from build123d import *

# Parameters (mm, degrees)
SKETCH_1_W          = 45
SKETCH_1_H          = 45
EXTRUDE_1_DEPTH     = 5
SKETCH_2_R          = 1
CUT_EXTRUDE_2_DEPTH = 5
SKETCH_3_W          = 35
SKETCH_3_H          = 5
CUT_EXTRUDE_3_DEPTH = 33.210246817
SKETCH_4_W          = 5
SKETCH_4_H          = 40
EXTRUDE_2_DEPTH     = 20


with BuildPart() as part:
    # 草圖1 → 填料-伸長1 (new body)
    with BuildSketch(Plane.XY):
        Rectangle(SKETCH_1_W, SKETCH_1_H)
    extrude(amount=EXTRUDE_1_DEPTH)

    # 草圖2 → 除料-伸長2 (cut)
    with BuildSketch(Plane(origin=(22.5, 0, 0), x_dir=(0, 0, -1), z_dir=(1, 0, 0))):
        with Locations(Location((-2.5, 20, 0), (0, 0, 90))):
            Circle(SKETCH_2_R)
    cut_extrude_2 = extrude(amount=-CUT_EXTRUDE_2_DEPTH, mode=Mode.SUBTRACT)

    # 草圖3 → 除料-伸長3 (cut, through all)
    with BuildSketch(Plane(origin=(0, 0, 0), x_dir=(-1, 0, 0), z_dir=(0, 0, -1))):
        with Locations((0, 20)):
            Rectangle(SKETCH_3_W, SKETCH_3_H)
    extrude(amount=-CUT_EXTRUDE_3_DEPTH, mode=Mode.SUBTRACT)

    # 鏡射1: 除料-伸長2 across plane
    add(cut_extrude_2.mirror(Plane(origin=(0, 0, 0), x_dir=(0, 0, 1), z_dir=(1, 0, 0))), mode=Mode.SUBTRACT)

    # 草圖4 → 填料-伸長2 (add)
    with BuildSketch(Plane(origin=(0, 0, 0), x_dir=(-1, 0, 0), z_dir=(0, 0, -1))):
        with Locations((-20, -2.5)):
            Rectangle(SKETCH_4_W, SKETCH_4_H)
    extrude_2 = extrude(amount=EXTRUDE_2_DEPTH)

    # 鏡射2: 填料-伸長2 across plane
    add(extrude_2.mirror(Plane(origin=(0, 0, 0), x_dir=(0, 0, 1), z_dir=(1, 0, 0))))


solid = part.part
Can you work these out from the model? Positions are in its coordinate system, mm. A direction names the side the tool comes from. Give positions to 0.01 mm unless a question says otherwise; leave off trailing zeros. Loops run counter-clockwise (first coordinate to the right, second up) from the corner with the lowest first, then second, coordinate; pieces in that order, holes last. Notation, with made-up numbers: (-28.5, -14) - (-16.5, -14) arc R37 cw to (-16.5, 25) - close; hole circle Ø1 at (38.5, -33.75). An arc over 180 degrees is marked (long way). Answer as a JSON object with one key per item and string values.
Q1. If I drill on L1, parallel to Z at x = -21, y = 20; L2, parallel to X at y = -18, z = -1.25; L3, parallel to Z at x = -12, y = -8.5, over which ranges is the centre line in solid material (lowest first)?
Geometry says:
{"L1": "0 to 1.5, 3.5 to 5", "L2": "-22.5 to -17.5, 17.5 to 22.5", "L3": "0 to 5"}
Q2. Imagine slicing it at D-D on y = -4. Write out the boundary of the cut face in (x, z).
Geometry says:
{"outline": "(-22.5, -20) - (-17.5, -20) - (-17.5, 0) - (17.5, 0) - (17.5, -20) - (22.5, -20) - (22.5, 5) - (-22.5, 5) - close"}
Q3. Will these pins go through, and if not, where does the flat tip stop? P1, Ø1.5, axis at x = -20, y = 20, coming from the -Z side; P2, Ø3, axis at y = 20, z = 2.5, coming from the +X side; P3, Ø5.5, axis at x = -3, z = 2, coming from the +Y side.
Geometry says:
{"P1": "z = 0", "P2": "x = 22.5", "P3": "y = 17.5"}
Q4. Imagine slicing it at B-B on y = 20. Write out the boundary of the cut face in (x, z).
Geometry says:
{"outline": "(-22.5, 0) - (-17.5, 0) - (-17.5, 1.5) - (-22.5, 1.5) - close; (-22.5, 3.5) - (-17.5, 3.5) - (-17.5, 5) - (-22.5, 5) - close; (17.5, 0) - (22.5, 0) - (22.5, 1.5) - (17.5, 1.5) - close; (17.5, 3.5) - (22.5, 3.5) - (22.5, 5) - (17.5, 5) - close"}
Q5. Imagine slicing it at C-C on z = -7.75. Write out the boundary of the cut face in (x, y), plus the area to 3 significant figures.
Geometry says:
{"outline": "(-22.5, -22.5) - (-17.5, -22.5) - (-17.5, 17.5) - (-22.5, 17.5) - close; (17.5, -22.5) - (22.5, -22.5) - (22.5, 17.5) - (17.5, 17.5) - close", "area": "400 mm²"}
Q6. Which directions (+Z, -Z, +X, -X, +Y, -Y) give clear straight access to the entire face, cutting with the end or side of a thin tool? Please do faces 1 (the flat face through (-17.5, 20, 1)), 2 (the flat face through (20, 20, 0)), 3 (the flat face through (17.5, -3, -10)).
Geometry says:
{"face 1": "+Z, -Z, +Y", "face 2": "-Z, +X, -X, +Y", "face 3": "-Z, +Y, -Y"}
Q7. Imagine slicing it at A-A on z = 2.5. Write out the boundary of the cut face in (x, y).
Geometry says:
{"outline": "(-22.5, -22.5) - (22.5, -22.5) - (22.5, 19) - (17.5, 19) - (17.5, 17.5) - (-17.5, 17.5) - (-17.5, 19) - (-22.5, 19) - close; (-22.5, 21) - (-17.5, 21) - (-17.5, 22.5) - (-22.5, 22.5) - close; (17.5, 21) - (22.5, 21) - (22.5, 22.5) - (17.5, 22.5) - close"}
Q8. If we mould it in two halves opening along X, with no side actions, what happens to faces 4 (the flat face through (0, -2, 0)), 5 (the flat face through (-20, -2, -20)), 6 (the flat face through (-22.5, 0, -7))? For each: pulls with the +X half, pulls with the -X half, needs draft (parallel to the pull), parting line crosses it, or undercut.
Geometry says:
{"face 4": "undercut", "face 5": "needs draft", "face 6": "pulls with the -X half"}
